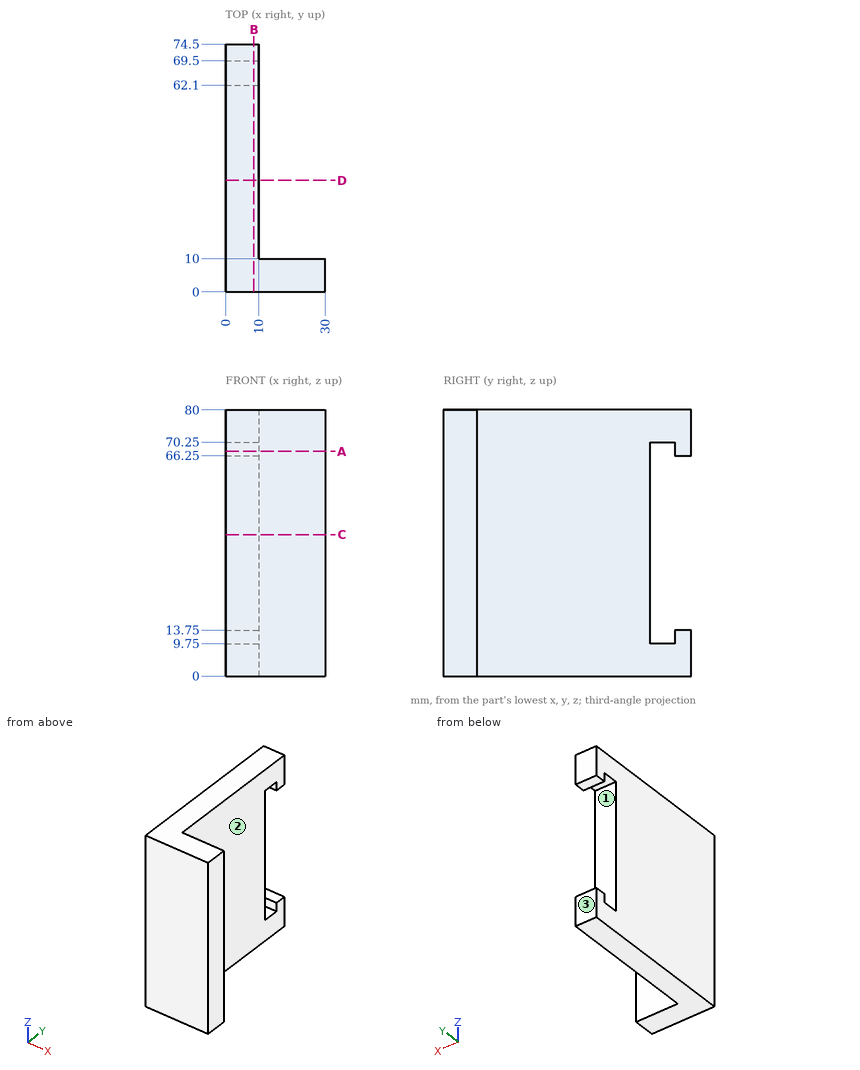
Design review of the part shown in the three views and the two pictorial views. Dimensions are in mm from the part's minimum x, y and z. A direction names the side the tool comes from. Round coordinates to 2 decimals unless told otherwise and drop trailing zeros. Write each loop counter-clockwise with the first axis right and the second up, starting at its lowest first coordinate (ties: lowest second). Pieces come first, ordered by that corner, then holes.
1) Machinability: for the marked faces 1, 2 and 3, which of the approach directions +Z, -Z, +X, -X, +Y, -Y give a long, thin tool a straight path to every point of the face, cutting with its end or side? Answer none if there is none.
Answer below:
face 1: +X, -X
face 2: +Z, -Z, +X, +Y
face 3: +Z, -Z, +X, -X, +Y
2) Insertion check: pin 1 Ø3 at (x, z) = (7, 12) entering from -Y; pin 2 Ø8 at (x, z) = (3, 29.5) entering from +Y; pin 3 Ø6 at (x, z) = (24.5, 18.5) entering from +Y; pin 4 Ø1 at (y, z) = (48.5, 30.5) entering from +X. Each pin has a flat end and moves straight along its axis. Give the tip position at first contact, or say it passes through.
Answer below:
pin 1: stops at y = 0
pin 2: stops at y = 62.1
pin 3: stops at y = 10
pin 4: stops at x = 10
3) Take a section at B-B on x = 8.5. Give the boundary of the cut face in (y, z).
Answer below:
outline: (0, 0) - (74.5, 0) - (74.5, 13.75) - (69.5, 13.75) - (69.5, 9.75) - (62.1, 9.75) - (62.1, 70.25) - (69.5, 70.25) - (69.5, 66.25) - (74.5, 66.25) - (74.5, 80) - (0, 80) - close
4) Take a section at C-C on z = 42.5. Give the boundary of the cut face in (x, y), then the cut area to 3 significant figures.
Answer below:
outline: (0, 0) - (30, 0) - (30, 10) - (10, 10) - (10, 62.1) - (0, 62.1) - close
area: 821 mm2
5) For line 1 along Y through (x, z) = (19.75, 70); line 2 along Y through (x, z) = (2, 19), list the stretches that pass through material, from the lowest coordinate up.
Answer below:
line 1: y = 0 to 10
line 2: y = 0 to 62.1
6) Take a section at A-A on z = 67.5. Give the boundary of the cut face in (x, y), then the cut area to 3 significant figures.
Answer below:
outline: (0, 0) - (30, 0) - (30, 10) - (10, 10) - (10, 62.1) - (0, 62.1) - close; (0, 69.5) - (10, 69.5) - (10, 74.5) - (0, 74.5) - close
area: 871 mm2
7) Take a section at D-D on y = 33.5. Give the boundary of the cut face in (x, z).
Answer below:
outline: (0, 0) - (10, 0) - (10, 80) - (0, 80) - close
